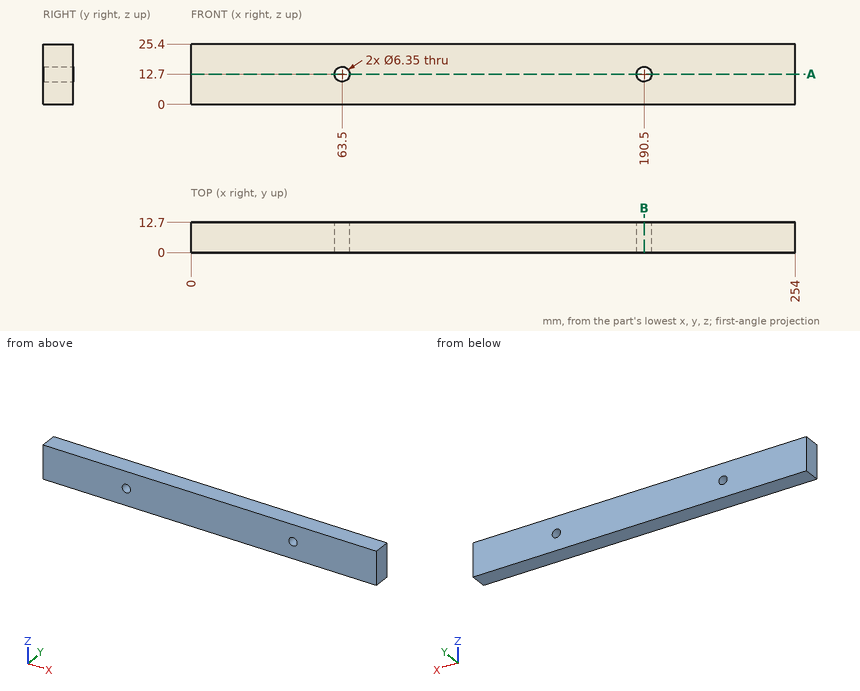
Input: dimensioned drawing with shaded views. Units: mm. Origin: part minimum x, y, z. Coordinates: 2 decimals unless noted, no trailing zeros. Loops run counter-clockwise (first coordinate to the right, second up) from the corner with the lowest first, then second, coordinate; pieces in that order, holes last.
Q1. Line query: line 1 along Z through (x, y) = (190.5, 6.75) (3 decimals); line 2 along X through (y, z) = (10, 15.5); line 3 along X through (y, z) = (9, 15). Output: solid intervals per line, ascending.
Results are:
line 1: z = 0 to 9.525, 15.875 to 25.4
line 2: x = 0 to 62, 65 to 189, 192 to 254
line 3: x = 0 to 61.31, 65.69 to 188.31, 192.69 to 254
Q2. Section B-B, the plane x = 190.5. Return the cut outline in (y, z) (3 decimals).
Results are:
outline: (0, 0) - (12.7, 0) - (12.7, 9.525) - (0, 9.525) - close; (0, 15.875) - (12.7, 15.875) - (12.7, 25.4) - (0, 25.4) - close
Q3. Section A-A, the plane z = 12.7. Return the cut outline in (x, y) (3 decimals), and give its area (3 significant figures).
Results are:
outline: (0, 0) - (60.325, 0) - (60.325, 12.7) - (0, 12.7) - close; (66.675, 0) - (187.325, 0) - (187.325, 12.7) - (66.675, 12.7) - close; (193.675, 0) - (254, 0) - (254, 12.7) - (193.675, 12.7) - close
area: 3,060 mm2
